Geometry check sheet. Reference: drawing and pictorial views, mm from the part's lowest x, y, z. A direction names the side the tool comes from. Give positions to 0.01 mm unless a question says otherwise; leave off trailing zeros. Order: outer loops, then holes, each group sorted by start corner. A loop starts at its lowest first (then second) coordinate and runs counter-clockwise, first axis right, second up. Notation, with made-up numbers: M 57,-29.75 L 94,-29.75 A14 cw 94,-23.75 Z; hole C 16,84 d1. An arc over 180 degrees is marked long. Answer as a JSON object with one key per item and string values. Group by question number.
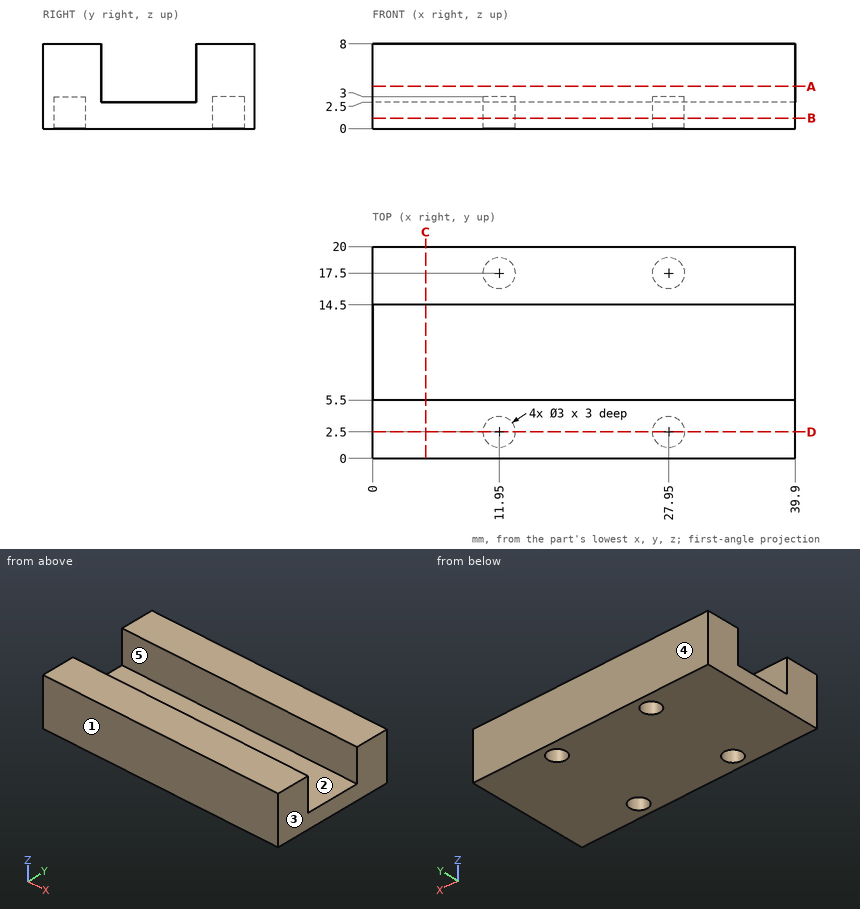
1. Cross-section at A-A (z = 4). Record the cut outline in (x, y).
2. Depth check by flat-ended pin: pin 1 (2.5 mm diameter, centred on x = 27.95, y = 2.5, fed in from -Z). Enter the tip coordinate at first touch or a pass-through.
3. Access from +Z, -Z, +X, -X, +Y, -Y to the whole of each face (thin tool, end or side, straight path). Record for the marked faces 4 and 5.
4. Cross-section at B-B (z = 1). Record the cut outline in (x, y).
5. Cross-section at D-D (y = 2.5). Record the cut outline in (x, z), and give its area (3 significant figures).
6. Thickness scan on line 1 along Y through (x, z) = (27.95, 2.1); line 2 along X through (y, z) = (2.5, 1.9); line 3 along Y through (x, z) = (10, 4). Record the ranges inside material, lowest first. Write a range as [from, to].
7. Cross-section at C-C (x = 5). Record the cut outline in (y, z), and give its area (4 significant figures).
8. Release check for a two-part mould opening along Y. For the marked faces 1, 2 and 3 record: released by +Y, released by -Y, zero draft, split by the parting line, or undercut.
Report:
{
 "1": {"outline": "M 0,0 L 39.9,0 L 39.9,5.5 L 0,5.5 Z; M 0,14.5 L 39.9,14.5 L 39.9,20 L 0,20 Z"},
 "2": {"pin 1": "stops at z = 3"},
 "3": {"face 4": "+Z, -Z, +X, -X, +Y", "face 5": "+Z, +X, -X"},
 "4": {"outline": "M 0,0 L 39.9,0 L 39.9,20 L 0,20 Z; hole C 11.95,2.5 d3; hole C 11.95,17.5 d3; hole C 27.95,2.5 d3; hole C 27.95,17.5 d3"},
 "5": {"outline": "M 0,0 L 10.45,0 L 10.45,3 L 13.45,3 L 13.45,0 L 26.45,0 L 26.45,3 L 29.45,3 L 29.45,0 L 39.9,0 L 39.9,8 L 0,8 Z", "area": "301 mm2"},
 "6": {"line 1": "y = [0, 1], [4, 16], [19, 20]", "line 2": "x = [0, 10.45], [13.45, 26.45], [29.45, 39.9]", "line 3": "y = [0, 5.5], [14.5, 20]"},
 "7": {"outline": "M 0,0 L 20,0 L 20,8 L 14.5,8 L 14.5,2.5 L 5.5,2.5 L 5.5,8 L 0,8 Z", "area": "110.5 mm2"},
 "8": {"face 1": "released by -Y", "face 2": "undercut", "face 3": "zero draft"}
}
